Could you check a few things on this model? Use its own coordinates, in mm. Face numbers are marked on the shaded views. A direction names the side the tool comes from. Coordinates: 2 decimals unless noted, no trailing zeros. Loops run counter-clockwise (first coordinate to the right, second up) from the corner with the lowest first, then second, coordinate; pieces in that order, holes last. Notation, with made-up numbers: M 13.25,63.25 L 22.25,63.25 A38 cw 22.25,101.25 Z; hole C 23,18 d4. An arc over 180 degrees is marked long. Return JSON: item names as keys, results as strings. Group by question number.
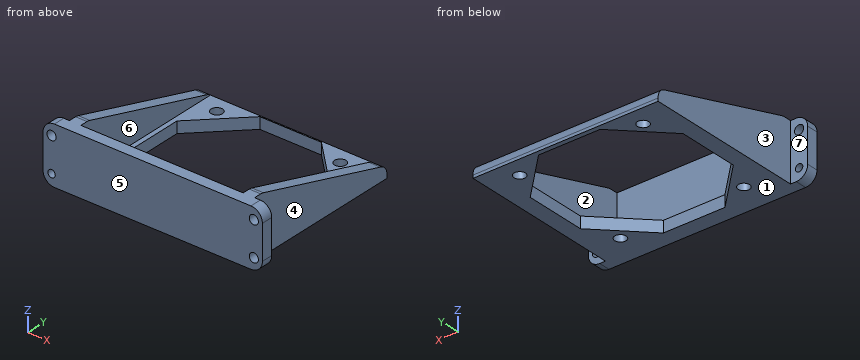
from build123d import *

# Parameters (mm, degrees)
SKETCH4_W                = 71
SKETCH4_H                = 71
SKETCH4_R                = 2.5
BOSS_EXTRUDE3_DEPTH      = 5
BOSS_EXTRUDE4_DEPTH      = 20
BOSS_EXTRUDE4_DEPTH_BACK = 5
CUT_EXTRUDE1_DEPTH       = 94.948123983
FILLET2_START            = -41
FILLET2_DEPTH            = 82
SKETCH8_W                = 7.5
SKETCH8_H                = 5
BOSS_EXTRUDE5_DEPTH      = 25
FILLET3_R                = 5
SKETCH10_R               = 2
SKETCH10_R_2             = 1.620466931
CUT_EXTRUDE2_DEPTH       = 25


with BuildPart() as part:
    # Sketch4 → Boss-Extrude3 (new body)
    with BuildSketch(Plane.XY):
        Rectangle(SKETCH4_W, SKETCH4_H)
        with Locations((-27, 27)):
            Circle(SKETCH4_R, mode=Mode.SUBTRACT)
        with Locations((27, 27)):
            Circle(SKETCH4_R, mode=Mode.SUBTRACT)
        with Locations((27, -27)):
            Circle(SKETCH4_R, mode=Mode.SUBTRACT)
        with Locations((-27, -27)):
            Circle(SKETCH4_R, mode=Mode.SUBTRACT)
        Polygon((-33.446601953, 13.48642712), (-13.48642712, 33.446601953), (13.48642712, 33.446601953), (33.446601953, 13.48642712), (33.446601953, -13.48642712), (13.48642712, -33.446601953), (-13.48642712, -33.446601953), (-33.446601953, -13.48642712), align=None, mode=Mode.SUBTRACT)
    extrude(amount=BOSS_EXTRUDE3_DEPTH)

    # Sketch5 → Boss-Extrude4 (add, two sides: drawn at the far end of the back side and taken through both)
    with BuildSketch(Plane.XY.offset(5).offset(-BOSS_EXTRUDE4_DEPTH_BACK)):
        Polygon((-35.5, 35.5), (-40.5, 35.5), (-40.5, -38.999937635), (-40.5, -40.5), (40.5, -40.5), (40.5, -38.999937635), (40.5, 35.5), (35.5, 35.5), (35.5, -35.5), (-35.5, -35.5), align=None)
    extrude(amount=BOSS_EXTRUDE4_DEPTH + BOSS_EXTRUDE4_DEPTH_BACK)

    # Sketch6 → Cut-Extrude1 (cut, through all)
    with BuildSketch(Plane.ZY.offset(40.5)):
        Polygon((5, 35.5), (25, 35.5), (25, -31.5), align=None)
    extrude(amount=-CUT_EXTRUDE1_DEPTH, mode=Mode.SUBTRACT)

    # Fillet2: read off the stored shape, not the designer's step
    # Fillet2 outline → Fillet2 (cut)
    with BuildSketch(Plane.YZ.offset(FILLET2_START)):
        with BuildLine():
            add(Edge.make_bspline(
                [(-30.800168474, 24.791095067), (-31.5, 25), (-32.230346106, 25)],
                knots=[0, 0, 0, 1, 1, 1], degree=2))
            Line((-30.800168474, 24.791095067), (-31.5, 25))
            Line((-31.5, 25), (-32.230346106, 25))
        make_face()
        with BuildLine():
            Line((35.5, 1.27452355), (35.5, 5))
            Line((35.5, 5), (31.930177632, 6.065618617))
            add(Edge.make_bspline(
                [(31.930177632, 6.065618617), (35.5, 5), (35.5, 1.27452355)],
                knots=[0.651540973, 0.651540973, 0.651540973, 1.651540973, 1.651540973, 1.651540973], degree=2))
        make_face()
    extrude(amount=FILLET2_DEPTH, mode=Mode.SUBTRACT)

    # Sketch8 → Boss-Extrude5 (add)
    with BuildSketch(Plane.XY.offset(25)):
        with Locations((-44.25, -38)):
            Rectangle(SKETCH8_W, SKETCH8_H)
        with Locations((44.25, -38)):
            Rectangle(SKETCH8_W, SKETCH8_H)
    extrude(amount=-BOSS_EXTRUDE5_DEPTH)

    # Fillet3
    fillet3_edges = [part.edges().sort_by_distance(p)[0] for p in [
        (-48, -38, 0),
        (-48, -38, 25),
        (48, -38, 0),
        (48, -38, 25),
    ]]
    fillet(fillet3_edges, radius=FILLET3_R)

    # Sketch10 → Cut-Extrude2 (cut)
    with BuildSketch(Plane(origin=(0, -35.5, 0), x_dir=(1, 0, 0), z_dir=(0, 1, 0))):
        with Locations(Location((44.25, -5, 0), (0, 0, 270))):
            Circle(SKETCH10_R)
        with Locations(Location((-44.25, -5, 0), (0, 0, 270))):
            Circle(SKETCH10_R_2)
        with Locations(Location((-44.25, -20, 0), (0, 0, 270))):
            Circle(SKETCH10_R)
        with Locations(Location((44.25, -20, 0), (0, 0, 270))):
            Circle(SKETCH10_R)
    extrude(amount=-CUT_EXTRUDE2_DEPTH, mode=Mode.SUBTRACT)


solid = part.part
(1) Imagine slicing it at B-B, the plane y = -19. Write out the boundary of the cut face in (x, z).
(2) Imagine slicing it at D-D, the plane z = 8.5. Write out the boundary of the cut face in (x, y) (3 decimals).
(3) We'd pull the mould along X, two halves only. Please class the marked faces 1, 2, 3 and 4: +X half, -X half, draft (parallel to the pull), parting line (faces both ways), or undercut.
(4) Imagine slicing it at C-C, the plane y = -27. Write out the boundary of the cut face in (x, z).
(5) Imagine slicing it at A-A, the plane x = -44.25. Write out the boundary of the cut face in (y, z).
(6) For the marked faces 5, 6 and 7, which set-ups out of +Z, -Z, +X, -X, +Y, -Y let a thin tool reach every point of the face, with its end or its side?
(7) Will these pins go through, and if not, where does the flat tip stop? P1, Ø4, axis at y = -2, z = 1.5, coming from the +X side; P2, Ø2.5, axis at y = 1, z = 1.5, coming from the -X side; P3, Ø3.5, axis at x = 44.25, z = 20, coming from the -Y side; P4, Ø10, axis at x = -22.5, z = 19, coming from the +Y side.
(8) If I drill on L1, parallel to X at y = -4, z = 12.25; L2, parallel to Y at x = -25, z = 1.75; L3, parallel to Z at x = -44, y = -38, over which ranges is the centre line in solid material (lowest first)? Write a range as [from, to].
Checks:
{
 "1": {"outline": "M -40.5,0 L -27.93,0 L -27.93,5 L -35.5,5 L -35.5,21.27 L -40.5,21.27 Z; M 27.93,0 L 40.5,0 L 40.5,21.27 L 35.5,21.27 L 35.5,5 L 27.93,5 Z"},
 "2": {"outline": "M -48,-40.5 L 48,-40.5 L 48,-35.5 L 40.5,-35.5 L 40.5,23.775 L 35.5,23.775 L 35.5,-35.5 L -35.5,-35.5 L -35.5,23.775 L -40.5,23.775 L -40.5,-35.5 L -48,-35.5 Z"},
 "3": {"face 1": "draft", "face 2": "undercut", "face 3": "-X half", "face 4": "+X half"},
 "4": {"outline": "M -40.5,0 L -29.5,0 L -29.5,5 L -35.5,5 L -35.5,23.66 L -40.5,23.66 Z; M -24.5,0 L -19.93,0 L -19.93,5 L -24.5,5 Z; M 19.93,0 L 24.5,0 L 24.5,5 L 19.93,5 Z; M 29.5,0 L 40.5,0 L 40.5,23.66 L 35.5,23.66 L 35.5,5 L 29.5,5 Z"},
 "5": {"outline": "M -40.5,0.16 L -35.5,0.16 L -35.5,3.38 L -40.5,3.38 Z; M -40.5,6.62 L -35.5,6.62 L -35.5,18 L -40.5,18 Z; M -40.5,22 L -35.5,22 L -35.5,24.84 L -40.5,24.84 Z"},
 "6": {"face 5": "+Z, -Z, +X, -X, -Y", "face 6": "+Z, +Y", "face 7": "+Z, -Z, -X, +Y"},
 "7": {"P1": "x = 40.5", "P2": "x = -40.5", "P3": "through", "P4": "y = -35.5"},
 "8": {"L1": "[-40.5, -35.5], [35.5, 40.5]", "L2": "[-40.5, -28.5], [-25.5, -21.93], [21.93, 25.5], [28.5, 35.48]", "L3": "[0.1, 3.4], [6.6, 18.02], [21.98, 24.9]"}
}
